The drawing under review shows one solid part. Ordinate dimensions are in mm from its lowest x, y, z. A direction names the side the tool comes from. Coordinates: 2 decimals unless noted, no trailing zeros. Write each loop counter-clockwise with the first axis right and the second up, starting at its lowest first coordinate (ties: lowest second). Pieces come first, ordered by that corner, then holes. Notation, with made-up numbers: (-38, 14.5) - (-11, 14.5) arc R17 cw to (-11, 31.5) - close; hole circle Ø7 at (21, -2.75). An arc over 180 degrees is marked (long way). Use a Markdown table: item, result.
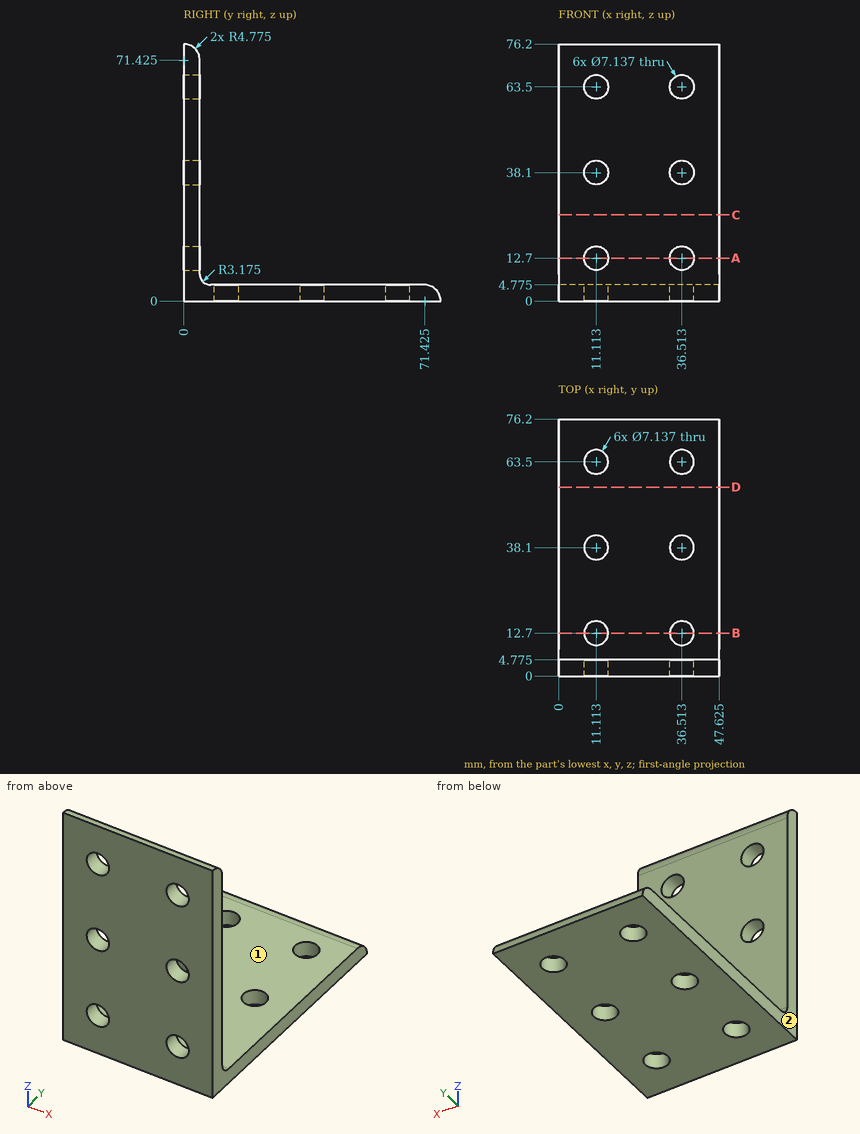
(1) For pin 1 (1.5 mm diameter, centred on x = 11, y = 43, fed in from -Z); pin 2 (2 mm diameter, centred on x = 42, y = 49, fed in from +Z) (1 decimal); pin 3 (4.5 mm diameter, centred on x = 36.51, y = 38.1, fed in from +Z); pin 4 (9.5 mm diameter, centred on x = 11.11, z = 38.1, fed in from +Y) (1 decimal), all flat-tipped, find the tip position at first contact; note any pin that passes through.
Determined:
| item | result |
|---|---|
| pin 1 | z = 0 |
| pin 2 | z = 4.8 |
| pin 3 | through |
| pin 4 | y = 4.8 |
(2) Take a section at A-A on z = 12.7. Write out the cut boundary in (x, y) (1 decimal), and give its area (3 significant figures).
Determined:
| item | result |
|---|---|
| outline | (0, 0) - (7.5, 0) - (7.5, 4.8) - (0, 4.8) - close; (14.7, 0) - (32.9, 0) - (32.9, 4.8) - (14.7, 4.8) - close; (40.1, 0) - (47.6, 0) - (47.6, 4.8) - (40.1, 4.8) - close |
| area | 159 mm2 |
(3) For L1, parallel to X at y = 38.1, z = 1.6 (1 decimal); L2, parallel to X at y = 12, z = 3 (1 decimal); L3, parallel to Z at x = 34.5, y = 52.5 (1 decimal), list the stretches that pass through material, from the lowest coordinate up. Write a range as from..to.
Determined:
| item | result |
|---|---|
| L1 | 0..7.5, 14.7..32.9, 40.1..47.6 |
| L2 | 0..7.6, 14.6..33, 40..47.6 |
| L3 | 0..4.8 |
(4) Take a section at C-C on z = 25.5. Write out the cut boundary in (x, y) (1 decimal).
Determined:
| item | result |
|---|---|
| outline | (0, 0) - (47.6, 0) - (47.6, 4.8) - (0, 4.8) - close |
(5) Machinability: for the marked faces 1 and 2, which of the approach directions +Z, -Z, +X, -X, +Y, -Y give a long, thin tool a straight path to every point of the face, cutting with its end or side? Answer none if there is none.
Determined:
| item | result |
|---|---|
| face 1 | +Z, +X, -X, +Y |
| face 2 | +Z, -Z, -X, +Y, -Y |
